Can you work these out from the drawing? Everything is in mm from the part's minimum corner. Round coordinates to 2 decimals unless told otherwise and drop trailing zeros. Loops run counter-clockwise (first coordinate to the right, second up) from the corner with the lowest first, then second, coordinate; pieces in that order, holes last. Notation, with made-up numbers: (0, 50.25) - (26, 50.25) arc R13 cw to (26, 71.25) - close; hole circle Ø5 at (7.5, -29). An arc over 180 degrees is marked (long way). Answer as a JSON object with one key per item and string values. Group by question number.
1) If I drill on line 1 along Z through (x, y) = (111, 25); line 2 along X through (y, z) = (35.5, 68), over which ranges is the centre line in solid material (lowest first)? Write a range as [from, to].
2) If we mould it in two halves opening along Z, with no side actions, what happens to the marked faces 1, 2 and 3? For each: pulls with the +Z half, pulls with the -Z half, needs draft (parallel to the pull), parting line crosses it, or undercut.
3) Will this pin go through, and if not, where does the flat tip stop? P1, Ø9.5, axis at y = 32, z = 59.5, coming from the +X side.
4) I want a section at B-B, the plane y = 22. Please give me the cut outline in (x, z).
5) I want a section at C-C, the plane z = 65.5. Please give me the cut outline in (x, y).
6) I want a section at A-A, the plane x = 103. Please give me the cut outline in (y, z).
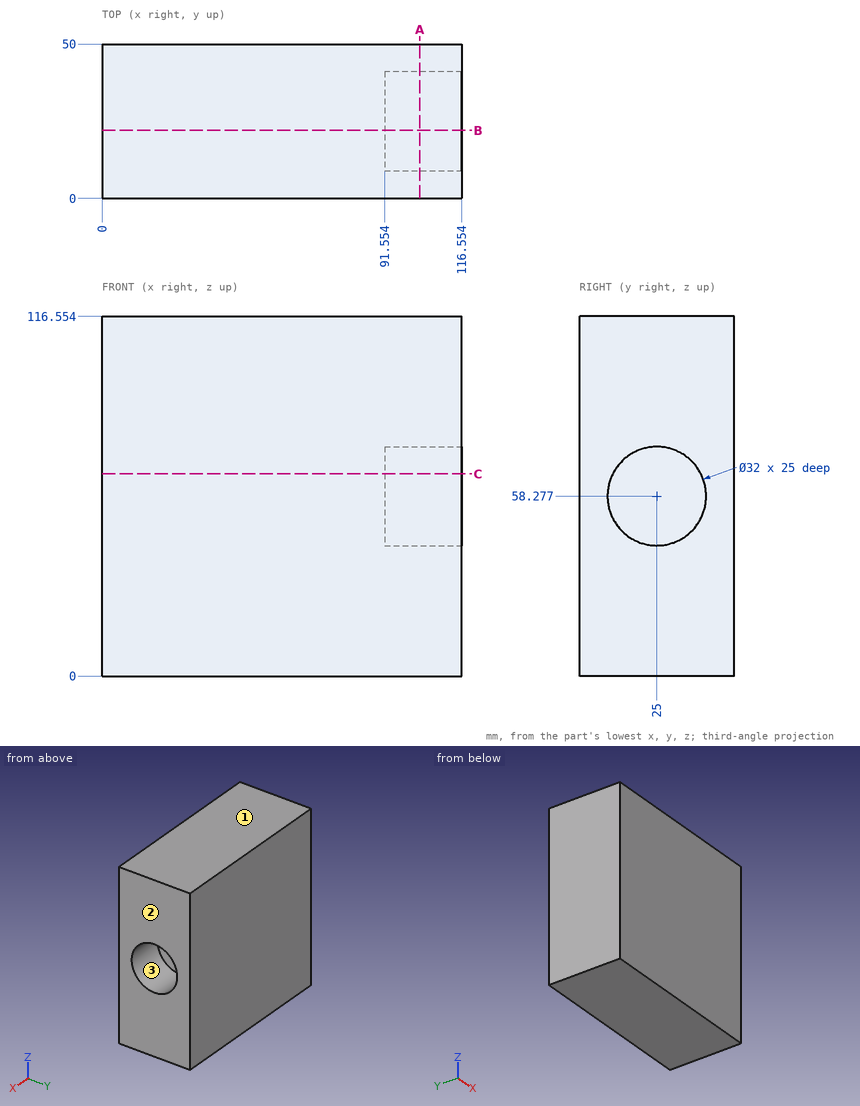
Outcome:
{
 "1": {"line 1": "[0, 42.28], [74.28, 116.55]", "line 2": "[0, 91.55]"},
 "2": {"face 1": "pulls with the +Z half", "face 2": "needs draft", "face 3": "undercut"},
 "3": {"P1": "x = 91.55"},
 "4": {"outline": "(0, 0) - (116.55, 0) - (116.55, 42.56) - (91.55, 42.56) - (91.55, 73.99) - (116.55, 73.99) - (116.55, 116.55) - (0, 116.55) - close"},
 "5": {"outline": "(0, 0) - (116.55, 0) - (116.55, 10.72) - (91.55, 10.72) - (91.55, 39.28) - (116.55, 39.28) - (116.55, 50) - (0, 50) - close"},
 "6": {"outline": "(0, 0) - (50, 0) - (50, 116.55) - (0, 116.55) - close; hole circle Ø32 at (25, 58.28)"}
}
